from build123d import *

# Parameters (mm, degrees)
SKETCH2_W           = 120
SKETCH2_H           = 45
BOSS_EXTRUDE2_DEPTH = 14
SHELL1_T            = -3


with BuildPart() as part:
    # Sketch2 → Boss-Extrude2 (new body)
    with BuildSketch(Plane.XY):
        Rectangle(SKETCH2_W, SKETCH2_H)
    extrude(amount=BOSS_EXTRUDE2_DEPTH)

    # Shell1
    shell1_openings = [part.faces().sort_by_distance(p)[0] for p in [
        (0, 0, 14),
    ]]
    offset(amount=SHELL1_T, openings=shell1_openings, kind=Kind.INTERSECTION)


solid = part.part
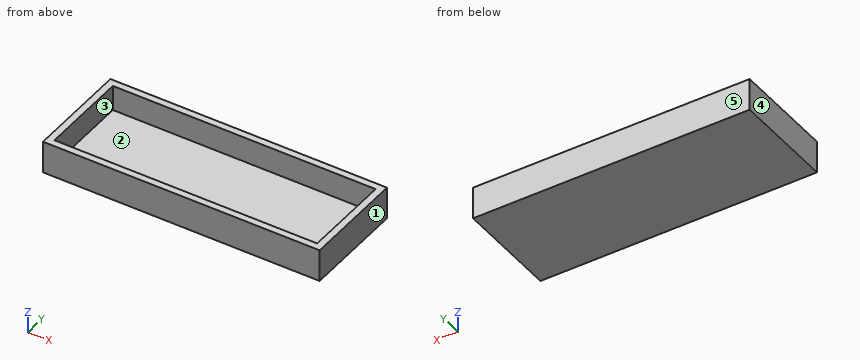
Here's how the part is built. I have some questions about the finished solid (model axes, mm). Face numbers are marked on the shaded views. A direction names the side the tool comes from. Coordinates: 2 decimals unless noted, no trailing zeros. Order: outer loops, then holes, each group sorted by start corner. A loop starts at its lowest first (then second) coordinate and runs counter-clockwise, first axis right, second up. Notation, with made-up numbers: M 12,-23 L 42,-23 A21 cw 42,-3 Z; hole C -27,80 d5. An arc over 180 degrees is marked long. Answer as CSV lines item,"result". Start each with the question number.
1. On a 3-axis mill with a long thin cutter (end or side, diameter ignored), from which of +Z, -Z, +X, -X, +Y, -Y can I reach the whole of each face in a straight line? I mean the marked faces 1 and 2. Say none if no direction works.
2. For pin 1 (11.5 mm diameter, centred on x = -17, y = -2, fed in from +Z); pin 2 (6 mm diameter, centred on x = -29.5, y = -9.5, fed in from -Z), each with a flat end and sliding along its axis, tell me the tip position at first contact or that it passes through.
3. We'd pull the mould along X, two halves only. Please class the marked faces 3, 4 and 5: released by +X, released by -X, zero draft, split by the parting line, or undercut.
4. I want a section at A-A, the plane y = 10. Write out the boundary of the cut face in (x, z).
5. I want a section at B-B, the plane z = 4.25. Write out the boundary of the cut face in (x, y), and give its area (3 significant figures).
6. I need wall thicknesses on line 1 (X direction, y = -9.5, z = 12.5); line 2 (Y direction, x = 37, z = 3.5); line 3 (Z direction, x = 49, y = -6). Which ranges of each line are inside material? Lowest first, please. Write a range as [from, to].
7. I want a section at C-C, the plane x = 31. Write out the boundary of the cut face in (y, z).
Recorded:
1,face 1,"+Z, -Z, +X, +Y, -Y"
1,face 2,"+Z"
2,pin 1,"stops at z = 3"
2,pin 2,"stops at z = 0"
3,face 3,"undercut"
3,face 4,"released by -X"
3,face 5,"zero draft"
4,outline,"M -60,0 L 60,0 L 60,14 L 57,14 L 57,3 L -57,3 L -57,14 L -60,14 Z"
5,outline,"M -60,-22.5 L 60,-22.5 L 60,22.5 L -60,22.5 Z; hole M -57,-19.5 L 57,-19.5 L 57,19.5 L -57,19.5 Z"
5,area,"954 mm2"
6,line 1,"x = [-60, -57], [57, 60]"
6,line 2,"y = [-22.5, -19.5], [19.5, 22.5]"
6,line 3,"z = [0, 3]"
7,outline,"M -22.5,0 L 22.5,0 L 22.5,14 L 19.5,14 L 19.5,3 L -19.5,3 L -19.5,14 L -22.5,14 Z"
